Study the drawing (mm; zero at the part's minimum x, y, z) and answer. A direction names the side the tool comes from. Coordinates: 2 decimals unless noted, no trailing zeros. Write each loop counter-clockwise with the first axis right and the second up, starting at its lowest first coordinate (ties: lowest second). Pieces come first, ordered by that corner, then holes. Notation, with made-up numbers: (-3.75, -6) - (9.25, -6) arc R32 cw to (9.25, 32) - close; hole circle Ø7 at (9.5, 11.25). An arc over 180 degrees is marked (long way). One line per item, written item: value.
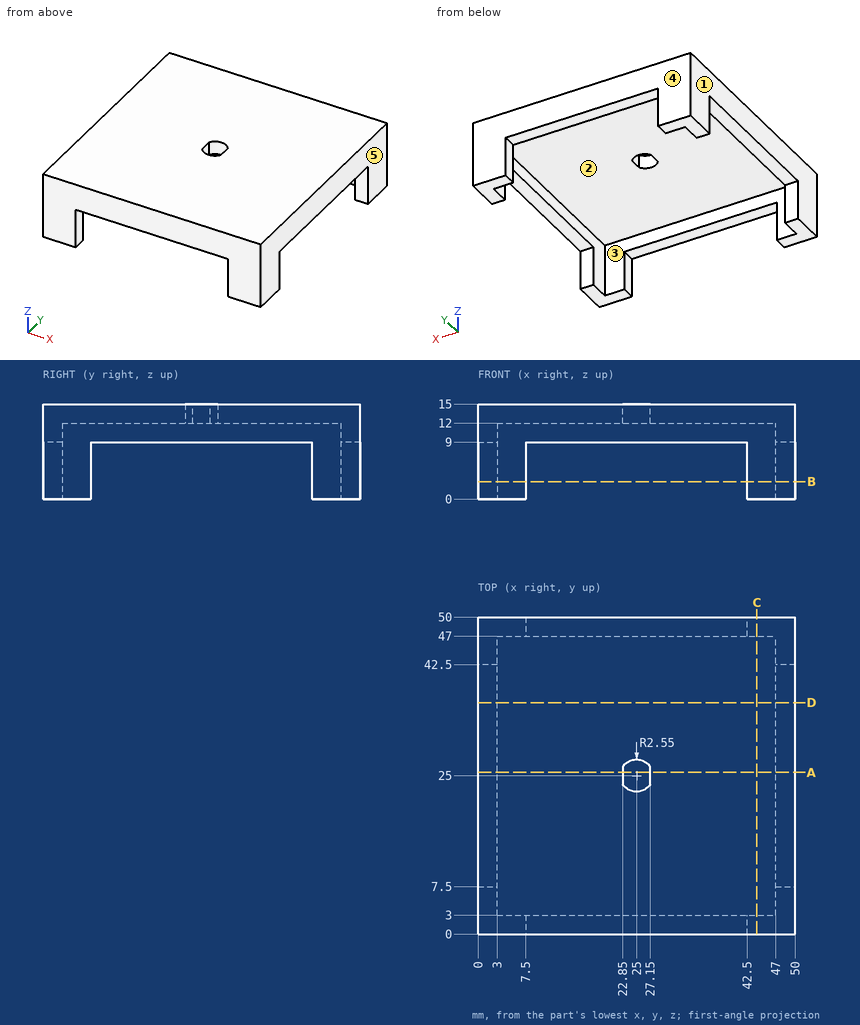
Item 1: Determine the mould class of the marked faces 3, 4 and 5 for opening direction Y: +Y half, -Y half, draft (parallel to the pull), parting line (faces both ways), or undercut.
Evaluation:
face 3: undercut
face 4: +Y half
face 5: draft
Item 2: Section C-C, the plane x = 44 is taken. Determine the outline of the cut face in (y, z), then the cut area to 3 significant figures.
Evaluation:
outline: (0, 0) - (3, 0) - (3, 12) - (47, 12) - (47, 0) - (50, 0) - (50, 15) - (0, 15) - close
area: 222 mm2
Item 3: Which of the six approach directions +Z, -Z, +X, -X, +Y, -Y give full straight-line access (tool end or side, diameter ignored) to the marked faces 1 and 2?
Evaluation:
face 1: +Z, -Z, -X, +Y, -Y
face 2: -Z
Item 4: Section D-D, the plane y = 36.5 is taken. Determine the outline of the cut face in (x, z), then the cut area to 3 significant figures.
Evaluation:
outline: (0, 9) - (3, 9) - (3, 12) - (47, 12) - (47, 9) - (50, 9) - (50, 15) - (0, 15) - close
area: 168 mm2
Item 5: Section B-B, the plane z = 2.75 is taken. Determine the outline of the cut face in (x, y), then the cut area to 3 significant figures.
Evaluation:
outline: (0, 0) - (7.5, 0) - (7.5, 3) - (3, 3) - (3, 7.5) - (0, 7.5) - close; (0, 42.5) - (3, 42.5) - (3, 47) - (7.5, 47) - (7.5, 50) - (0, 50) - close; (42.5, 0) - (50, 0) - (50, 7.5) - (47, 7.5) - (47, 3) - (42.5, 3) - close; (42.5, 47) - (47, 47) - (47, 42.5) - (50, 42.5) - (50, 50) - (42.5, 50) - close
area: 144 mm2
Item 6: Given pin 1 (6 mm diameter, centred on y = 15.5, z = 10.5, fed in from -X); pin 2 (5 mm diameter, centred on x = 24, y = 11, fed in from -Z); pin 3 (2.5 mm diameter, centred on x = 1.5, y = 30, fed in from -Z), each flat-ended and moving along its own axis, determine where each tip first touches the part or whether it passes through.
Evaluation:
pin 1: stops at x = 0
pin 2: stops at z = 12
pin 3: stops at z = 9
Item 7: Consider probe 1 along Y at (x, z) = (25, 12.5); probe 2 along Y at (x, z) = (38.5, 11.5); probe 3 along Z at (x, y) = (37.5, 28.5). Determine where each line is inside the solid, lowest interval first.
Evaluation:
probe 1: y = 0 to 22.45, 27.55 to 50
probe 2: y = 0 to 3, 47 to 50
probe 3: z = 12 to 15
Item 8: Section A-A, the plane y = 25.5 is taken. Determine the outline of the cut face in (x, z), then the cut area to 3 significant figures.
Evaluation:
outline: (0, 9) - (3, 9) - (3, 12) - (22.85, 12) - (22.85, 15) - (0, 15) - close; (27.15, 12) - (47, 12) - (47, 9) - (50, 9) - (50, 15) - (27.15, 15) - close
area: 155 mm2
